Part model, mm, in its own coordinate system. A direction names the side the tool comes from. Round coordinates to 2 decimals unless told otherwise and drop trailing zeros. Write each loop counter-clockwise with the first axis right and the second up, starting at its lowest first coordinate (ties: lowest second). Pieces come first, ordered by that corner, then holes.
Autodesk Inventor part; units mm, degrees
ref_plane "YZ Plane" through (0, 0, 0) normal (1, 0, 0) x (0, 1, 0)
ref_plane "XZ Plane" through (0, 0, 0) normal (0, 1, 0) x (-1, 0, 0)
ref_plane "XY Plane" through (0, 0, 0) normal (0, 0, 1) x (1, 0, 0)
sketch "Sketch1" plane through (0, 0, 0) normal (0, 1, 0) x (-1, 0, 0)
  circle A0 centre (0, 0) radius 11.049
  circle A1 centre (0, 0) radius 3.175
  circle A2 centre (8.025, 0) radius 1.5
  line L0 (9.525, 0) -> (11.049, 0)
  circle A3 centre (0, 0) radius 5.08
  circle A4 centre (0, 8.025) radius 1.5
  circle A5 centre (-8.025, 0) radius 1.5
  circle A6 centre (0, -8.025) radius 1.5
  point P0 (0, 9.525)
  point P1 (-9.525, 0)
  point P2 (0, -9.525)
  dimension "d0" = 22.098
  dimension "d2" = 3
  dimension "d1" = 6.35
  dimension "d3" = 1.524
  dimension "d4" = 10.16
  dimension "d7" = 360
extrude "Extrusion1" add sketch "Sketch1" along normal blind 3.81 contours A0 | A3
sketch "Sketch2" plane through (0, 3.81, 0) normal (0, 1, 0) x (1, 0, 0)
  circle A0 centre (0, 0) radius 5.08
  circle A1 centre (0, 0) radius 3.175
  dimension "d11" = 10.16
extrude "Extrusion2" add sketch "Sketch2" along normal blind 1.651
sketch "Sketch3" plane through (0, 0, 0) normal (0, -1, 0) x (1, 0, 0)
  circle A0 centre (0, 0) radius 5.08
  circle A1 centre (0, 0) radius 5.08
  circle A2 centre (0, 0) radius 3.175
extrude "Extrusion3" add sketch "Sketch3" along normal blind 10.16
thread "Thread1"
properties part number "Threaded Rod Mount"
Q1. Two-plate mould, pull along Z, no slides. Class faces 1 (the cylindrical face through (0.2, 1.88, -9.51)), 2 (the cylindrical face through (1.438, 1.878, -10.955)), 3 (the flat face through (-5, 0, -2)): released by +Z, released by -Z, zero draft, split by the parting line, or undercut.
Q2. Drop flat-ended pins along their axis: P1, Ø4, axis at x = -8.5, z = -5.5, coming from the -Y side; P2, Ø8, axis at x = 5.5, y = -2, coming from the -Z side; P3, Ø4, axis at x = -8.025, z = 0, coming from the +Y side; P4, Ø5, axis at x = 0, z = 0, coming from the +Y side. Give the stop position or say it passes through.
Q3. Saw through at C-C, the plane x = -7.25. Write the cut outline in (y, z).
Q4. Saw through at D-D, the plane z = 9. Write the cut outline in (x, y).
Q5. Saw through at A-A, the plane z = 0. Write the cut outline in (x, y) (3 decimals), and give its area (3 significant figures).
Q6. Saw through at B-B, the plane x = 0. Write the cut outline in (y, z) (3 decimals).
Q7. Tool access for faces 4 (the cylindrical face through (6.639, 1.878, 0.575)), 5 (the cylindrical face through (-0.661, -5.009, -5.037)), 6 (the flat face through (-5, 3.81, -2)): list every direction of +Z, -Z, +X, -X, +Y, -Y with a clear straight run to the whole face (end or side of a thin tool).
Q8. Wall check: line 1 (Z direction, x = 0, y = 1.35) (3 decimals); line 2 (Z direction, x = 0, y = -6) (3 decimals); line 3 (Y direction, x = 9.75, z = 1.25). Give the ranges that are in metal, low to high.
Computed:
1. face 1: undercut
1. face 2: split by the parting line
1. face 3: zero draft
2. P1: stops at y = 0
2. P2: stops at z = -10.86
2. P3: stops at y = 3.81
2. P4: passes through
3. outline: (0, -8.34) - (3.81, -8.34) - (3.81, -1.28) - (0, -1.28) - close; (0, 1.28) - (3.81, 1.28) - (3.81, 8.34) - (0, 8.34) - close
4. outline: (-6.41, 0) - (-1.14, 0) - (-1.14, 3.81) - (-6.41, 3.81) - close; (1.14, 0) - (6.41, 0) - (6.41, 3.81) - (1.14, 3.81) - close
5. outline: (-11.049, 0) - (-9.525, 0) - (-9.525, 3.81) - (-11.049, 3.81) - close; (-6.525, 0) - (-5.08, 0) - (-5.08, -10.16) - (-3.175, -10.16) - (-3.175, 5.461) - (-5.08, 5.461) - (-5.08, 3.81) - (-6.525, 3.81) - close; (3.175, -10.16) - (5.08, -10.16) - (5.08, 0) - (6.525, 0) - (6.525, 3.81) - (5.08, 3.81) - (5.08, 5.461) - (3.175, 5.461) - close; (9.525, 0) - (11.049, 0) - (11.049, 3.81) - (9.525, 3.81) - close
5. area: 82.1 mm2
6. outline: (-10.16, -5.08) - (0, -5.08) - (0, -6.525) - (3.81, -6.525) - (3.81, -5.08) - (5.461, -5.08) - (5.461, -3.175) - (-10.16, -3.175) - close; (-10.16, 3.175) - (5.461, 3.175) - (5.461, 5.08) - (3.81, 5.08) - (3.81, 6.525) - (0, 6.525) - (0, 5.08) - (-10.16, 5.08) - close; (0, -11.049) - (3.81, -11.049) - (3.81, -9.525) - (0, -9.525) - close; (0, 9.525) - (3.81, 9.525) - (3.81, 11.049) - (0, 11.049) - close
7. face 4: +Y, -Y
7. face 5: -Y
7. face 6: +Y
8. line 1: z = -11.049 to -9.525, -6.525 to -3.175, 3.175 to 6.525, 9.525 to 11.049
8. line 2: z = -5.08 to -3.175, 3.175 to 5.08
8. line 3: y = 0 to 3.81
